Check sheet for the modelled part. Datum: model origin and axes. Units: mm. Face numbers are marked on the shaded views. A direction names the side the tool comes from. Give positions to 0.01 mm unless a question says otherwise; leave off trailing zeros. Write each loop counter-clockwise with the first axis right and the second up, starting at its lowest first coordinate (ties: lowest second). Pieces come first, ordered by that corner, then holes. Notation, with made-up numbers: (72.5, 53.5) -> (131.5, 53.5) arc R26 cw to (131.5, 69.5) -> close; hole circle Ø11 at (68.5, -14). An arc over 180 degrees is marked (long way). Use a Markdown table: item, result. Add a question column.
1. Cross-section at A-A (z = 12). Enter the section's corners in (x, y), then the cut area to 3 significant figures.
2. Cross-section at B-B (x = 14). Enter the section's corners in (y, z).
3. Release check for a two-part mould opening along X. For the marked faces 3, 4 and 5 record: released by +X, released by -X, zero draft, split by the parting line, or undercut.
4. Cross-section at C-C (y = 26). Enter the section's corners in (x, z), then the cut area to 3 significant figures.
5. Cross-section at D-D (y = 15). Enter the section's corners in (x, z).
6. Gauge pin test, flat ends, axial feed: P1, Ø2, axis at y = 23.5, z = 1, coming from the -X side; P2, Ø10, axis at x = 9, z = 11.5, coming from the -Y side; P3, Ø6.5, axis at x = 14, y = 26, coming from the -Z side; P4, Ø4, axis at x = 13, y = 10.5, coming from the +Z side. Record the tip position at first contact, or that the pin passes through.
7. Set-up check for the marked faces 1 and 2: record each of +Z, -Z, +X, -X, +Y, -Y from which the full face is reachable in a straight line by a thin tool's end or side.
8. Scan lines: probe 1 along Y at (x, z) = (14, 0.5); probe 2 along Z at (x, y) = (12.25, 17); probe 3 along X at (y, z) = (18.75, 2.5). Record each from-to range of solid material in increasing order. Write a range as [from, to].
from build123d import *

# Parameters (mm, degrees)
F1_DEPTH = 30
F2_R     = 2.5
F3_DEPTH = 3
F4_R     = 6
F4_R_2   = 2.5
F5_DEPTH = 4
F6_R     = 2
F7_D     = 4
F7_DEPTH = 15
F7_TIP   = 1.2017212381


with BuildPart() as f1:
    # F0 (on Front) → F1 (new body)
    with BuildSketch(Plane.XZ):
        Polygon((0, 1), (0, 0), (28, 0), (28, 1), (28, 16), (27, 16), (27, 1), (1, 1), (1, 16), (0, 16), align=None)
    extrude(amount=-F1_DEPTH)

    # F2 (on face) → F3 (join)
    with BuildSketch(Plane.XY.offset(1)):
        with Locations((14, 15)):
            Circle(F2_R)
    extrude(amount=-F3_DEPTH)

    # F4 (on face) → F5 (join)
    with BuildSketch(Plane(origin=(0, 0, -2), x_dir=(1, 0, 0), z_dir=(0, 0, -1))):
        with Locations((14, -15)):
            Circle(F4_R)
        with Locations((14, -15)):
            Circle(F4_R_2, mode=Mode.SUBTRACT)
        with Locations((14, -15)):
            Circle(F4_R_2)
    extrude(amount=F5_DEPTH)

    # F6
    f6_edges = [f1.edges().sort_by_distance(p)[0] for p in [
        (27.5, 0, 16),
        (27.5, 30, 16),
        (0.5, 30, 16),
        (0.5, 0, 16),
    ]]
    fillet(f6_edges, radius=F6_R)

    # F7
    with Locations(Plane.XY.offset(1)):
        with Locations((14, 4), (14, 26)):
            Hole(F7_D / 2, depth=F7_DEPTH)
            with Locations((0, 0, -(F7_DEPTH + F7_TIP / 2))):  # 118° drill point
                Cone(0, F7_D / 2, F7_TIP, mode=Mode.SUBTRACT)


solid = f1.part
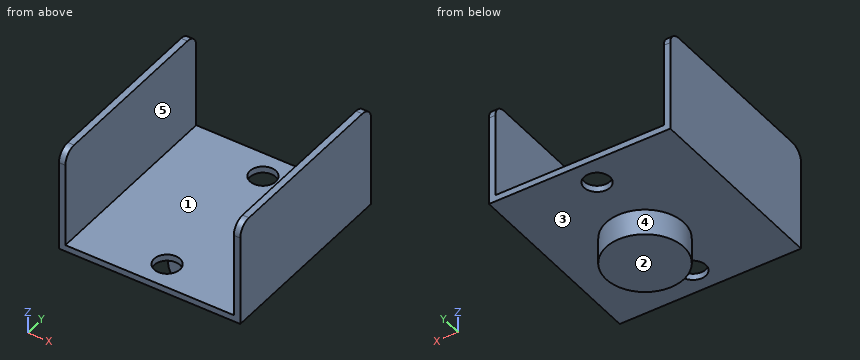
Worked answers:
| question | item | result |
|---|---|---|
| 1 | outline | (0, 0) -> (1, 0) -> (1, 30) -> (0, 30) -> close; (27, 0) -> (28, 0) -> (28, 30) -> (27, 30) -> close |
| 1 | area | 60.0 mm² |
| 2 | outline | (0, 0) -> (2, 0) -> (2, 1) -> (0, 1) -> close; (6, 0) -> (12.5, 0) -> (12.5, -2) -> (9, -2) -> (9, -6) -> (21, -6) -> (21, -2) -> (17.5, -2) -> (17.5, 0) -> (24, 0) -> (24, 1) -> (6, 1) -> close; (28, 0) -> (30, 0) -> (30, 1) -> (28, 1) -> close |
| 3 | face 3 | zero draft |
| 3 | face 4 | split by the parting line |
| 3 | face 5 | undercut |
| 4 | outline | (0, 0) -> (12, 0) -> (12, 1) -> (1, 1) -> (1, 16) -> (0, 16) -> close; (16, 0) -> (28, 0) -> (28, 16) -> (27, 16) -> (27, 1) -> (16, 1) -> close |
| 4 | area | 54.0 mm² |
| 5 | outline | (0, 0) -> (11.5, 0) -> (11.5, -2) -> (8, -2) -> (8, -6) -> (20, -6) -> (20, -2) -> (16.5, -2) -> (16.5, 0) -> (28, 0) -> (28, 16) -> (27, 16) -> (27, 1) -> (1, 1) -> (1, 16) -> (0, 16) -> close |
| 6 | P1 | stops at x = 0 |
| 6 | P2 | passes through |
| 6 | P3 | stops at z = 0 |
| 6 | P4 | stops at z = 1 |
| 7 | face 1 | +Z, +Y, -Y |
| 7 | face 2 | -Z, +X, -X, +Y, -Y |
| 8 | probe 1 | y = [0, 2], [6, 24], [28, 30] |
| 8 | probe 2 | z = [-6, -2], [0, 1] |
| 8 | probe 3 | x = [0, 1], [27, 28] |
